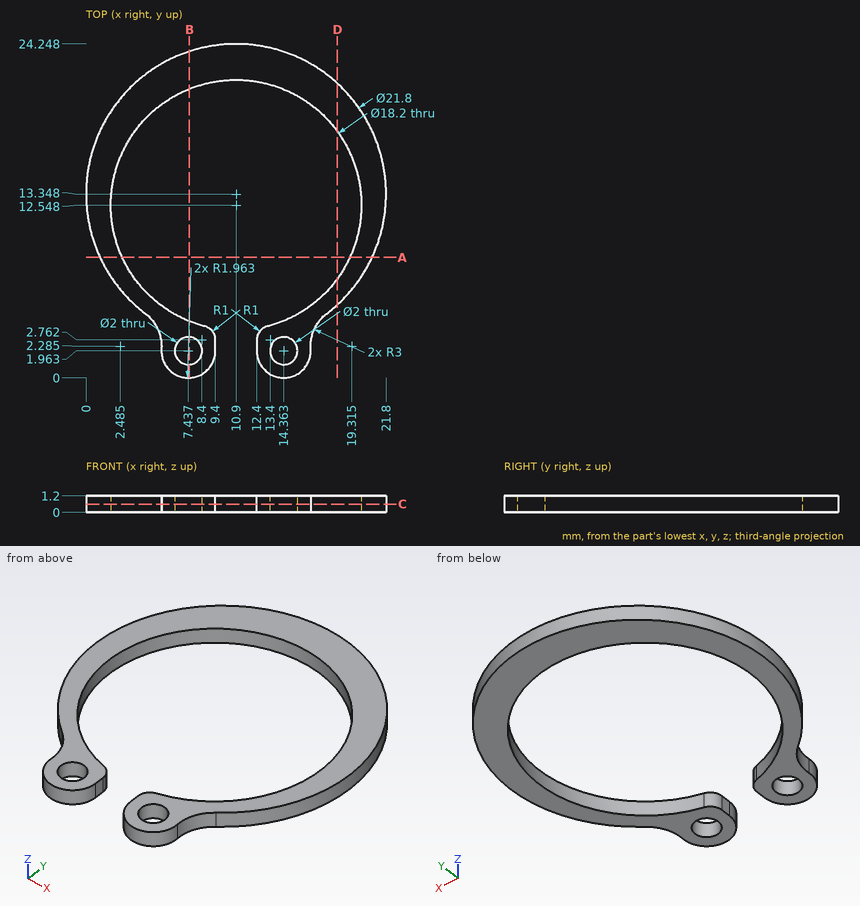
Answer from the drawing. Dimensions are ordinates in mm from the lowest x, y and z of the part. Round coordinates to 2 decimals unless told otherwise and drop trailing zeros. Write each loop counter-clockwise with the first axis right and the second up, starting at its lowest first coordinate (ties: lowest second). Pieces come first, ordered by that corner, then holes. Notation, with made-up numbers: (64.5, 3) - (114.5, 3) arc R9 cw to (114.5, 11) - close; hole circle Ø7 at (-19.75, 10). An arc over 180 degrees is marked (long way). Use a Markdown table: item, result.
(1) The part is cut by section D-D (x = 18.25). Write down the section's boundary in (y, z).
Reported:
| item | result |
|---|---|
| outline | (5.3, 0) - (7.18, 0) - (7.18, 1.2) - (5.3, 1.2) - close; (17.91, 0) - (21.4, 0) - (21.4, 1.2) - (17.91, 1.2) - close |
(2) The part is cut by section A-A (y = 8.75). Write down the section's boundary in (x, z).
Reported:
| item | result |
|---|---|
| outline | (1.02, 0) - (2.63, 0) - (2.63, 1.2) - (1.02, 1.2) - close; (19.17, 0) - (20.78, 0) - (20.78, 1.2) - (19.17, 1.2) - close |
(3) The part is cut by section B-B (x = 7.5). Write down the section's boundary in (y, z) (1 decimal).
Reported:
| item | result |
|---|---|
| outline | (0, 0) - (1, 0) - (1, 1.2) - (0, 1.2) - close; (3, 0) - (4.1, 0) - (4.1, 1.2) - (3, 1.2) - close; (21, 0) - (23.7, 0) - (23.7, 1.2) - (21, 1.2) - close |
(4) Straight lines are drawn through the part: line 1 along Y through (x, z) = (13.75, 0.2) (1 decimal); line 2 along Y through (x, z) = (14.25, 0.4) (1 decimal); line 3 along X through (y, z) = (20, 0.1) (1 decimal). For each, find the intervals that lie inside material, in ascending order. Write a range as [from, to].
Reported:
| item | result |
|---|---|
| line 1 | [0.1, 1.2], [2.8, 3.9], [21.2, 23.9] |
| line 2 | [0, 1], [3, 4.1], [21, 23.7] |
| line 3 | [2.3, 5.7], [16.1, 19.5] |
(5) Each of these flat-tipped pins is pushed along its axis until it touches: pin 1 Ø3 at (x, y) = (7.44, 1.96) entering from +Z; pin 2 Ø1 at (x, y) = (5, 18.5) entering from -Z; pin 3 Ø0.6 at (y, z) = (2.5, 1) entering from +X. Where does it stop, or does it pass through?
Reported:
| item | result |
|---|---|
| pin 1 | z = 1.2 |
| pin 2 | through |
| pin 3 | x = 16.36 |
(6) The part is cut by section C-C (z = 0.6). Write down the section's boundary in (x, y) (1 decimal), then the cut area to 3 significant figures.
Reported:
| item | result |
|---|---|
| outline | (4.3, 4.7) arc R3 cw to (5.5, 2.1) arc R2 ccw (long way) to (9.4, 2) - (9.4, 2.8) arc R1 ccw to (8.6, 3.7) arc R9.1 cw (long way) to (13.2, 3.7) arc R1 ccw to (12.4, 2.8) - (12.4, 2) arc R2 ccw (long way) to (16.3, 2.1) arc R3 cw to (17.5, 4.7) arc R10.9 ccw (long way) to start; hole circle Ø2 at (7.4, 2); hole circle Ø2 at (14.4, 2) |
| area | 125 mm2 |
